The listing builds one solid part. Answer for the finished solid, in the listing's coordinates (mm). A direction names the side the tool comes from. Round coordinates to 2 decimals unless told otherwise and drop trailing zeros. Loops run counter-clockwise (first coordinate to the right, second up) from the corner with the lowest first, then second, coordinate; pieces in that order, holes last. Notation, with made-up numbers: (-28.75, 77) -> (6.25, 77) arc R5 ccw to (6.25, 81) -> close; hole circle Ø7 at (8.25, 25.25). An arc over 180 degrees is marked (long way). One line per question, with ' | ' between items.
from build123d import *

# Parameters (mm, degrees)
SKETCH2_R               = 8.398
BOSS_EXTRUDE3_DEPTH     = 38.1
SKETCH2_3_R             = 9.525
SKETCH2_3_R_2           = 8.398
BOSS_EXTRUDE4_DEPTH     = 3.175
SKETCH3_R               = 6.35
CUT_EXTRUDE1_DEPTH      = 41.411152545
CUT_EXTRUDE1_DEPTH_BACK = 41.411152545
FILLET1_R               = 1.27


with BuildPart() as part:
    # Sketch2 → Boss-Extrude3 (new body)
    with BuildSketch(Plane.XY.offset(25.4)):
        with Locations(Location((0, 0, 0), (0, 0, 180))):
            Circle(SKETCH2_R)
    extrude(amount=BOSS_EXTRUDE3_DEPTH)


with BuildPart() as body_2:
    # Sketch2_3 → Boss-Extrude4 (new body)
    with BuildSketch(Plane.XY.offset(25.4)):
        Circle(SKETCH2_3_R)
        with Locations(Location((0, 0, 0), (0, 0, 180))):
            Circle(SKETCH2_3_R_2, mode=Mode.SUBTRACT)
        with Locations(Location((0, 0, 0), (0, 0, 180))):
            Circle(SKETCH2_3_R_2)
    extrude(amount=-BOSS_EXTRUDE4_DEPTH)


with BuildPart() as cut_extrude1_tool:
    # Sketch3 → Cut-Extrude1 (new, two sides)
    with BuildSketch(Plane.XY.offset(25.4)) as cut_extrude1_sk:
        Circle(SKETCH3_R)
    extrude(amount=CUT_EXTRUDE1_DEPTH)
    extrude(cut_extrude1_sk.sketch, amount=-CUT_EXTRUDE1_DEPTH_BACK)


with BuildPart() as part_1:
    add(part.part)

    # Cut-Extrude1: cut by cut_extrude1_tool
    add(cut_extrude1_tool.part, mode=Mode.SUBTRACT)


with BuildPart() as body_2_1:
    add(body_2.part)

    # Cut-Extrude1: cut by cut_extrude1_tool
    add(cut_extrude1_tool.part, mode=Mode.SUBTRACT)

    # Combine1: union part
    add(part_1.part)

    # Fillet1
    fillet1_edges = [body_2_1.edges().sort_by_distance(p)[0] for p in [
        (-6.35, 0, 22.225),
        (-9.525, 0, 22.225),
    ]]
    fillet(fillet1_edges, radius=FILLET1_R)


solid = body_2_1.part
Q1. A cutting plane is placed at A-A on x = 0. Give the vertices of the cut face in (y, z) (3 decimals).
Numbers:
outline: (-9.525, 23.495) arc R1.27 ccw to (-8.255, 22.225) -> (-7.62, 22.225) arc R1.27 ccw to (-6.35, 23.495) -> (-6.35, 63.5) -> (-8.398, 63.5) -> (-8.398, 25.4) -> (-9.525, 25.4) -> close; (6.35, 23.495) arc R1.27 ccw to (7.62, 22.225) -> (8.255, 22.225) arc R1.27 ccw to (9.525, 23.495) -> (9.525, 25.4) -> (8.398, 25.4) -> (8.398, 63.5) -> (6.35, 63.5) -> close
Q2. For a pull along X with two mould halves and no side action, classify faces 3 (the face through (-1.38, -6.2, 43.78)), 4 (the face through (-7.559, -5.796, 24.461)), 5 (the face through (5, -7, 25.4)) as pulls with the +X half, pulls with the -X half, needs draft (parallel to the pull), parting line crosses it, or undercut.
Numbers:
face 3: undercut | face 4: parting line crosses it | face 5: needs draft
Q3. Find the intervals of material crossed by line 1 (Y direction, x = 0, z = 45.5); line 2 (X direction, y = -0.25, z = 33.5); line 3 (X direction, y = 2.5, z = 32), in increasing order. Write a range as from..to.
Numbers:
line 1: -8.4..-6.35, 6.35..8.4 | line 2: -8.39..-6.35, 6.35..8.39 | line 3: -8.02..-5.84, 5.84..8.02
Q4. For faces 1 (the face through (5.5, -5.5, 22.225)), 2 (the face through (8.39, -0.37, 44.18)), determine the directions among +Z, -Z, +X, -X, +Y, -Y from which every point of the face is accessible in a straight line to the end or side of a thin tool.
Numbers:
face 1: -Z, +X, -X, +Y, -Y | face 2: +Z
Q5. A cutting plane is placed at C-C on z = 42.5. Give the vertices of the cut face in (x, y).
Numbers:
outline: circle Ø16.8 at (0, 0); hole circle Ø12.7 at (0, 0)
Q6. Given pin 1 Ø2 at (x, z) = (-7.5, 54) entering from +Y; pin 2 Ø1.5 at (x, z) = (7, 38.5) entering from -Y; pin 3 Ø8 at (x, z) = (-1, 38) entering from -Y; pin 4 Ø8 at (x, y) = (7.5, 6) entering from -Z (3 decimals), each flat-ended and moving along its own axis, determine where each tip first touches the part or whether it passes through.
Numbers:
pin 1: y = 5.32 | pin 2: y = -5.61 | pin 3: y = -8.4 | pin 4: z = 22.225
